Can you work these out from the model? Positions are in its coordinate system, mm. Give positions to 0.01 mm unless a question says otherwise; leave off trailing zeros. Order: outer loops, then holes, each group sorted by start corner. A loop starts at its lowest first (then second) coordinate and runs counter-clockwise, first axis right, second up. Notation, with made-up numbers: (62.5, 38.25) - (92.5, 38.25) arc R29 ccw to (92.5, 64.25) - close; hole circle Ø8 at (14, 46). An arc over 180 degrees is marked (long way). Use one line per item in the form item = value. Start each with the question number.
1) Suppose I cut it at B-B, the plane x = 0.6. Write out the boundary of the cut face in (y, z).
2) Suppose I cut it at C-C, the plane y = 8. Write out the boundary of the cut face in (x, z).
3) Please list where these lines run through material, in increasing order: probe 1 along Y at (x, z) = (-1.3, -1.1); probe 2 along Z at (x, y) = (0.1, 8.5); probe 3 along X at (y, z) = (3, -1.75).
4) Suppose I cut it at A-A, the plane z = -0.6. Write out the boundary of the cut face in (x, y), and give its area (3 significant figures).
```python
from build123d import *

# Parameters (mm, degrees)
SKETCH1_R           = 2
BOSS_EXTRUDE1_DEPTH = 33.5
SKETCH2_W           = 0.5
SKETCH2_H           = 0.2


with BuildPart() as part:
    # Sketch1 → Boss-Extrude1 (new body)
    with BuildSketch(Plane(origin=(0, 0, 0), x_dir=(1, 0, 0), z_dir=(0, 1, 0))):
        with Locations(Location((0, 0, 0), (0, 0, 270))):
            Circle(SKETCH1_R)
    extrude(amount=BOSS_EXTRUDE1_DEPTH)

    # Sketch2 → Cut-Revolve1 (revolve, cut)
    with BuildSketch(Plane.XY, mode=Mode.PRIVATE) as cut_revolve1_sk:
        with Locations((1.75, 0.9)):
            Rectangle(SKETCH2_W, SKETCH2_H)
    revolve(cut_revolve1_sk.sketch.rotate(Axis((0, -1.7, 0), (0, 1, 0)), 90), axis=Axis((0, -1.7, 0), (0, 1, 0)), mode=Mode.SUBTRACT)


solid = part.part
```
Result sheet:
q1.outline = (0, -1.91) - (0.8, -1.91) - (0.8, -1.37) - (1, -1.37) - (1, -1.91) - (33.5, -1.91) - (33.5, 1.91) - (1, 1.91) - (1, 1.37) - (0.8, 1.37) - (0.8, 1.91) - (0, 1.91) - close
q2.outline = circle Ø4 at (0, 0)
q3.probe_1 = 0 to 0.8, 1 to 33.5
q3.probe_2 = -2 to 2
q3.probe_3 = -0.97 to 0.97
q4.outline = (-1.91, 0) - (1.91, 0) - (1.91, 0.8) - (1.37, 0.8) - (1.37, 1) - (1.91, 1) - (1.91, 33.5) - (-1.91, 33.5) - (-1.91, 1) - (-1.37, 1) - (-1.37, 0.8) - (-1.91, 0.8) - close
q4.area = 128 mm²
